```python
from build123d import *

# Parameters (mm, degrees)
SKETCH1_W           = 1.5875
SKETCH1_H           = 177.8
BOSS_EXTRUDE1_DEPTH = 330.2
CUT_EXTRUDE1_DEPTH  = 1.5875
FILLET1_R           = 6.35


with BuildPart() as part:
    # Sketch1 → Boss-Extrude1 (new body)
    with BuildSketch(Plane(origin=(0, 0, 0), x_dir=(1, 0, 0), z_dir=(0, 1, 0))):
        with Locations((0.79375, 88.9)):
            Rectangle(SKETCH1_W, SKETCH1_H)
    extrude(amount=BOSS_EXTRUDE1_DEPTH)

    # Sketch2 → Cut-Extrude1 (cut)
    with BuildSketch(Plane.ZY):
        Polygon((-177.8, 50.8), (0, 330.2), (-177.8, 330.2), align=None)
    extrude(amount=-CUT_EXTRUDE1_DEPTH, mode=Mode.SUBTRACT)

    # Fillet1
    fillet1_edges = [part.edges().sort_by_distance(p)[0] for p in [
        (0.79375, 50.8, -177.8),
        (0.79375, 330.2, 0),
        (0.79375, 0, -177.8),
        (0.79375, 0, 0),
    ]]
    fillet(fillet1_edges, radius=FILLET1_R)


solid = part.part
```
Build history of the part. All positions in model axes, mm. Give positions to 0.01 mm unless a question says otherwise; leave off trailing zeros. Loops run counter-clockwise (first coordinate to the right, second up) from the corner with the lowest first, then second, coordinate; pieces in that order, holes last.
Item 1: Drill centre lines: line 1 (Z direction, x = 0.25, y = 205); line 2 (Y direction, x = 0.35, z = -68); line 3 (Y direction, x = 0.2, z = -34.5). Where is each one in solid material? Low to high.
Answers follow:
line 1: z = -79.67 to 0
line 2: y = 0 to 223.34
line 3: y = 0 to 275.99
Item 2: Slice it at A-A, the plane x = 0.9. List the corners of the cut face in (y, z), and give its area (3 significant figures).
Answers follow:
outline: (0, -171.45) arc R6.35 ccw to (6.35, -177.8) - (48.95, -177.8) arc R6.35 ccw to (52.36, -176.81) - (311.8, -11.71) arc R6.35 ccw to (308.39, 0) - (6.35, 0) arc R6.35 ccw to (0, -6.35) - close
area: 33,800 mm2
Item 3: Slice it at C-C, the plane y = 201.5. List the corners of the cut face in (x, z), and give its area (3 significant figures).
Answers follow:
outline: (0, -81.9) - (1.59, -81.9) - (1.59, 0) - (0, 0) - close
area: 130 mm2
Item 4: Slice it at B-B, the plane z = -35. List the corners of the cut face in (x, y).
Answers follow:
outline: (0, 0) - (1.59, 0) - (1.59, 275.2) - (0, 275.2) - close
